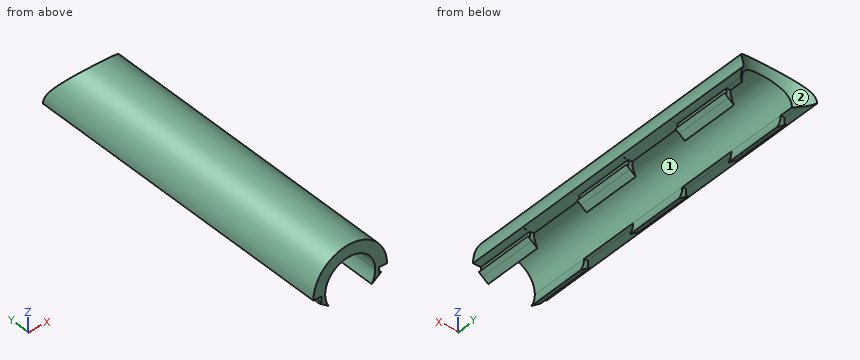
Autodesk Inventor part; units mm, degrees
ref_plane "Work Plane2" through (0.0017, -6.74, -2) normal (0, 1, 0) x (-1, 0, 0)
ref_plane "Work Plane3" through (0, 0, -8) normal (0, 0, -1) x (-1, 0.0001, 0)
ref_plane "YZ Plane" through (0, 0, 0) normal (1, 0, 0) x (0, 1, 0)
ref_plane "Work Plane2" through (0.0017, -6.74, -2) normal (0, 1, 0) x (-1, 0, 0)
sketch "Sketch1" plane through (0.0017, -6.74, -2) normal (0, 1, 0) x (-1, 0, 0)
  line L0 (-2.7483, 0) -> (0, 0) construction
  line L1 (0, 0) -> (0.0017, 6)
  line L2 (1.7517, 6) -> (-1.7483, 6) construction
  arc A0 (-3.9294, 1.3826) -> (-4.2492, 3) centre (0.0008, 3) ccw construction
  arc A1 (-3.413, 0.4685) -> (3.4132, 0.4666) centre (0.0008, 3) ccw construction
  line L3 (5.1396, 2.9983) -> (6.2508, 2.9983)
  arc A2 (-6.2492, 3.0017) -> (6.2508, 2.9983) centre (0.0008, 3) ccw construction
  line L4 (5.7129, 2.1908) -> (5.1396, 2.1908) construction
  line L5 (5.1396, 2.1908) -> (5.1396, 2.9983) construction
  line L6 (-5.138, 3.0011) -> (-6.2492, 3.0017)
  line L7 (-5.7117, 2.194) -> (-5.1384, 2.1937) construction
  line L8 (-5.1384, 2.1937) -> (-5.138, 3.0011) construction
  line L9 (5.7129, 2.1908) -> (3.4132, 0.4666) construction
  line L10 (-5.7117, 2.194) -> (-3.413, 0.4685) construction
  line L11 (5.1396, 2.5258) -> (4.8896, 2.5258) construction
  line L12 (5.1396, 2.1908) -> (5.1396, 2.0408) construction
  line L13 (4.7148, 1.4425) -> (4.6248, 1.5625) construction
  line L14 (5.2628, 2.0408) -> (4.6248, 1.5625)
  line L15 (5.2628, 2.0408) -> (4.8896, 2.0408)
  line L16 (5.1396, 2.9983) -> (4.8896, 2.9983)
  line L17 (4.8896, 2.0408) -> (4.8896, 2.9983)
  line L18 (4.6248, 1.5625) -> (3.6609, 0.8398)
  arc A3 (3.6609, 0.8398) -> (4.2508, 2.9983) centre (0.0008, 3) ccw
  line L19 (-5.2617, 2.0437) -> (-4.624, 1.5651)
  line L20 (-5.2617, 2.0437) -> (-4.8885, 2.0435)
  line L21 (-5.138, 3.0011) -> (-4.888, 3.001)
  line L22 (-4.8885, 2.0435) -> (-4.888, 3.001)
  line L23 (-4.624, 1.5651) -> (-3.6604, 0.8418)
  arc A4 (-4.2492, 3.0006) -> (-3.6604, 0.8418) centre (0.0008, 3) ccw
  arc A5 (4.2508, 2.9983) -> (-4.2492, 3.0006) centre (0.0008, 3) ccw
  arc A6 (-6.2492, 3.0017) -> (6.2508, 2.9983) centre (0.0008, 3) ccw construction
  arc A7 (6.2508, 2.9983) -> (-6.2492, 3.0017) centre (0.0008, 3) ccw
  point P0 (0.0017, 2)
  point P1 (3.9302, 1.3805)
  dimension "d0" = 8.5
  dimension "d3" = 12.5
extrude "Extrusion4" add sketch "Sketch1" against normal blind 50.8
ref_plane "Work Plane3" through (0, 0, -8) normal (0, 0, -1) x (-1, 0.0001, 0)
sketch "Sketch2" plane through (0, 0, -8) normal (0, 0, -1) x (-1, 0.0001, 0)
  circle A0 centre (0, 0) radius 6.74
extrude "Extrusion5" add sketch "Sketch1" along normal blind 5
extrude "Extrusion6" cut sketch "Sketch2" against normal blind 100
sketch "Sketch3" plane through (4.8902, -57.54, 0.0435) normal (1, 0, 0.0006) x (0.0006, 0, -1)
  line L0 (-0.0029, 0) -> (1.199, 0)
  line L1 (1.199, 0) -> (1.2011, 10) construction
  line L2 (1.2011, 51.8817) -> (1.2011, 0)
  line L3 (1.2011, 10) -> (1.2011, 20)
  line L4 (1.2011, 20) -> (1.2011, 30) construction
  line L5 (1.2011, 30) -> (1.2011, 40)
  line L6 (1.2011, 40) -> (1.2011, 50) construction
  line L7 (-0.9574, 55.0191) -> (-0.9574, 0)
  line L8 (1.2011, 50) -> (-0.9574, 50)
  line L9 (-0.9574, 50) -> (-0.9574, 55.0191)
  line L10 (-0.9574, 55.0191) -> (1.2011, 55.0191)
  line L11 (1.2011, 55.0191) -> (1.2011, 50)
  line L12 (-0.9601, 52.8994) -> (-0.9601, 0)
  line L13 (1.2011, 40) -> (-0.9601, 40)
  line L14 (-0.9601, 40) -> (-0.9601, 30)
  line L15 (-0.9601, 30) -> (1.2011, 30)
  line L16 (1.2011, 30) -> (1.2011, 40)
  line L17 (1.2011, 20) -> (-0.9601, 20)
  line L18 (-0.9601, 20) -> (-0.9601, 10)
  line L19 (-0.9601, 10) -> (1.2011, 10)
  line L20 (1.2011, 10) -> (1.2011, 20)
  point P0 (0.0408, 57.54)
  dimension "d27" = 10
  dimension "d28" = 10
  dimension "d29" = 10
  dimension "d30" = 10
  dimension "d31" = 10
extrude "Extrusion7" cut sketch "Sketch3" along normal mid plane 100 contours L2 L8 L7 L10 L11 | L2 L15 L7 L13 | L7 L15 L12 L13 | L2 L19 L7 L17 | L7 L19 L12 L17
properties part number "drone motor arm top"
Verification items for the finished model (mm, model axes). Face numbers are marked on the shaded views. A direction names the side the tool comes from. Coordinates: 2 decimals unless noted, no trailing zeros. Loops run counter-clockwise (first coordinate to the right, second up) from the corner with the lowest first, then second, coordinate; pieces in that order, holes last. Notation, with made-up numbers: (68.25, -34) -> (119.25, -34) arc R22 ccw to (119.25, -11) -> close; hole circle Ø4 at (70.25, 30.25). An arc over 180 degrees is marked (long way). Put each result on its own line as item: value.
1. Section check B-B, the plane z = 1.5. Record the boundary of the cut face in (x, y), then the cut area to 3 significant figures.
Result set:
outline: (-6.23, -57.54) -> (-4.22, -57.54) -> (-4.22, -5.26) arc R6.74 cw to (-6.23, -2.57) -> close; (4.22, -57.54) -> (6.23, -57.54) -> (6.23, -2.57) arc R6.74 cw to (4.22, -5.25) -> close
area: 215 mm^2
2. Section check C-C, the plane y = -9. Record the boundary of the cut face in (x, z).
Result set:
outline: (-6.25, 1) -> (-4.89, 1) -> (-4.89, 0.04) -> (-5.26, 0.04) -> (-4.62, -0.44) -> (-3.66, -1.16) arc R4.25 cw to (-4.25, 1) arc R4.25 cw to (4.25, 1) arc R4.25 cw to (3.66, -1.16) -> (4.63, -0.43) -> (5.26, 0.04) -> (4.89, 0.04) -> (4.89, 1) -> (5.14, 1) -> (6.25, 1) arc R6.25 ccw to start
3. Thickness scan on line 1 (Y direction, x = 5, z = 0); line 2 (X direction, y = -17, z = 1.5); line 3 (X direction, y = -6, z = 6.25). Record the ranges inside material, lowest first.
Result set:
line 1: y = -57.54 to -47.54, -37.54 to -27.54, -17.54 to -7.54
line 2: x = -6.23 to -4.22, 4.22 to 6.23
line 3: x = -3.39 to -3.07, 3.07 to 3.39
4. Tool access check on the marked faces 1 and 2. Record the directions out of +Z, -Z, +X, -X, +Y, -Y that give a thin tool (end or side, any length) a straight path to the whole face; none if there is none.
Result set:
face 1: +Y, -Y
face 2: +Z, -Z, +Y
5. Section check D-D, the plane z = 6.25. Record the boundary of the cut face in (x, y).
Result set:
outline: (-3.39, -57.54) -> (3.39, -57.54) -> (3.39, -5.82) arc R6.74 cw to (-3.39, -5.83) -> close
6. Gauge pin test, flat ends, axial feed: P1, Ø1.7, axis at x = 5, z = -0.5, coming from the +Y side; P2, Ø4, axis at x = 2.5, z = 1, coming from the -Y side; P3, Ø5, axis at y = -35, z = 6, coming from the +X side; P4, Ø1, axis at x = -4, y = -42, coming from the +Z side. Record the tip position at first contact, or that the pin passes through.
Result set:
P1: stops at y = -7.54
P2: stops at y = -57.54
P3: stops at x = 5.73
P4: stops at z = 6.18
